```python
from build123d import *

# Parameters (mm, degrees)
SKETCH1_W           = 48
SKETCH1_H           = 53
BOSS_EXTRUDE1_DEPTH = 10
SKETCH2_W           = 48
SKETCH2_H           = 5.616325
BOSS_EXTRUDE2_DEPTH = 33.1917878
SKETCH4_W           = 4
SKETCH4_H           = 10
BOSS_EXTRUDE4_DEPTH = 40
SKETCH5_W           = 48
SKETCH5_H           = 10.8609375
BOSS_EXTRUDE5_DEPTH = 23.1917878
SKETCH6_W           = 48
SKETCH6_H           = 5
BOSS_EXTRUDE6_DEPTH = 42.3
SKETCH7_W           = 12.8082122
SKETCH7_H           = 16.4772625
BOSS_EXTRUDE7_DEPTH = 48
CUT_EXTRUDE1_REACH  = 84.426
SKETCH8_R           = 11.5
SKETCH8_R_2         = 2
FILLET1_R           = 10
FILLET2_R           = 4
SKETCH9_W           = 5
SKETCH9_H           = 16.4772625
BOSS_EXTRUDE9_DEPTH = 48


with BuildPart() as part:
    # Sketch1 → Boss-Extrude1 (new body)
    with BuildSketch(Plane.XY):
        with Locations((24, 26.5)):
            Rectangle(SKETCH1_W, SKETCH1_H)
    extrude(amount=BOSS_EXTRUDE1_DEPTH)

    # Sketch2 → Boss-Extrude2 (add)
    with BuildSketch(Plane(origin=(0, 0, 0), x_dir=(-1, 0, 0), z_dir=(0, 0, -1))):
        with Locations((-24, -2.8081625)):
            Rectangle(SKETCH2_W, SKETCH2_H)
    extrude(amount=-BOSS_EXTRUDE2_DEPTH)

    # Sketch4 → Boss-Extrude4 (add)
    with BuildSketch(Plane.XY.offset(10)):
        with Locations((2, 48)):
            Rectangle(SKETCH4_W, SKETCH4_H)
        with Locations((46, 48)):
            Rectangle(SKETCH4_W, SKETCH4_H)
    extrude(amount=BOSS_EXTRUDE4_DEPTH)

    # Sketch5 → Boss-Extrude5 (add)
    with BuildSketch(Plane.XY.offset(10)):
        with Locations((24, 5.43046875)):
            Rectangle(SKETCH5_W, SKETCH5_H)
    extrude(amount=BOSS_EXTRUDE5_DEPTH)

    # Sketch6 → Boss-Extrude6 (add)
    with BuildSketch(Plane.XZ.offset(5.616325)):
        with Locations((24, 30.6917878)):
            Rectangle(SKETCH6_W, SKETCH6_H)
    extrude(amount=BOSS_EXTRUDE6_DEPTH)

    # Sketch7 → Boss-Extrude7 (add)
    with BuildSketch(Plane.ZY):
        with Locations((-6.4041061, 2.62230625)):
            Rectangle(SKETCH7_W, SKETCH7_H)
    extrude(amount=-BOSS_EXTRUDE7_DEPTH)

    # Sketch8 → Cut-Extrude1 (cut, up to next)
    with BuildSketch(Plane(origin=(0, 0, 28.1917878), x_dir=(-1, 0, 0), z_dir=(0, 0, -1)), mode=Mode.PRIVATE) as cut_extrude1_sk1:
        with Locations((-24, -26.616325)):
            Circle(SKETCH8_R)
    cut_extrude1_tool1 = extrude(cut_extrude1_sk1.sketch, amount=-CUT_EXTRUDE1_REACH, mode=Mode.PRIVATE) & part.part
    # Sketch8 → Cut-Extrude1 (cut, up to next)
    with BuildSketch(Plane(origin=(0, 0, 28.1917878), x_dir=(-1, 0, 0), z_dir=(0, 0, -1)), mode=Mode.PRIVATE) as cut_extrude1_sk2:
        with Locations((-39.5, -11.116325)):
            Circle(SKETCH8_R_2)
    cut_extrude1_tool2 = extrude(cut_extrude1_sk2.sketch, amount=-CUT_EXTRUDE1_REACH, mode=Mode.PRIVATE) & part.part
    # Sketch8 → Cut-Extrude1 (cut, up to next)
    with BuildSketch(Plane(origin=(0, 0, 28.1917878), x_dir=(-1, 0, 0), z_dir=(0, 0, -1)), mode=Mode.PRIVATE) as cut_extrude1_sk3:
        with Locations((-39.5, -42.116325)):
            Circle(SKETCH8_R_2)
    cut_extrude1_tool3 = extrude(cut_extrude1_sk3.sketch, amount=-CUT_EXTRUDE1_REACH, mode=Mode.PRIVATE) & part.part
    # Sketch8 → Cut-Extrude1 (cut, up to next)
    with BuildSketch(Plane(origin=(0, 0, 28.1917878), x_dir=(-1, 0, 0), z_dir=(0, 0, -1)), mode=Mode.PRIVATE) as cut_extrude1_sk4:
        with Locations((-8.5, -11.116325)):
            Circle(SKETCH8_R_2)
    cut_extrude1_tool4 = extrude(cut_extrude1_sk4.sketch, amount=-CUT_EXTRUDE1_REACH, mode=Mode.PRIVATE) & part.part
    # Sketch8 → Cut-Extrude1 (cut, up to next)
    with BuildSketch(Plane(origin=(0, 0, 28.1917878), x_dir=(-1, 0, 0), z_dir=(0, 0, -1)), mode=Mode.PRIVATE) as cut_extrude1_sk5:
        with Locations((-8.5, -42.116325)):
            Circle(SKETCH8_R_2)
    cut_extrude1_tool5 = extrude(cut_extrude1_sk5.sketch, amount=-CUT_EXTRUDE1_REACH, mode=Mode.PRIVATE) & part.part
    add(cut_extrude1_tool1.solids().sort_by_distance((24, -26.616325, 28.191788))[0], mode=Mode.SUBTRACT)
    add(cut_extrude1_tool2.solids().sort_by_distance((39.5, -11.116325, 28.191788))[0], mode=Mode.SUBTRACT)
    add(cut_extrude1_tool3.solids().sort_by_distance((39.5, -42.116325, 28.191788))[0], mode=Mode.SUBTRACT)
    add(cut_extrude1_tool4.solids().sort_by_distance((8.5, -11.116325, 28.191788))[0], mode=Mode.SUBTRACT)
    add(cut_extrude1_tool5.solids().sort_by_distance((8.5, -42.116325, 28.191788))[0], mode=Mode.SUBTRACT)

    # Fillet1
    fillet1_edges = [part.edges().sort_by_distance(p)[0] for p in [
        (24, 10.8609375, 0),
    ]]
    fillet(fillet1_edges, radius=FILLET1_R)

    # Fillet2
    fillet2_edges = [part.edges().sort_by_distance(p)[0] for p in [
        (2, 43, 10),
        (46, 43, 10),
    ]]
    fillet(fillet2_edges, radius=FILLET2_R)

    # Sketch9 → Boss-Extrude9 (add)
    with BuildSketch(Plane(origin=(48, 0, 0), x_dir=(0, 0, -1), z_dir=(1, 0, 0))):
        with Locations((15.3082122, 2.62230625)):
            Rectangle(SKETCH9_W, SKETCH9_H)
    extrude(amount=-BOSS_EXTRUDE9_DEPTH)


solid = part.part
```
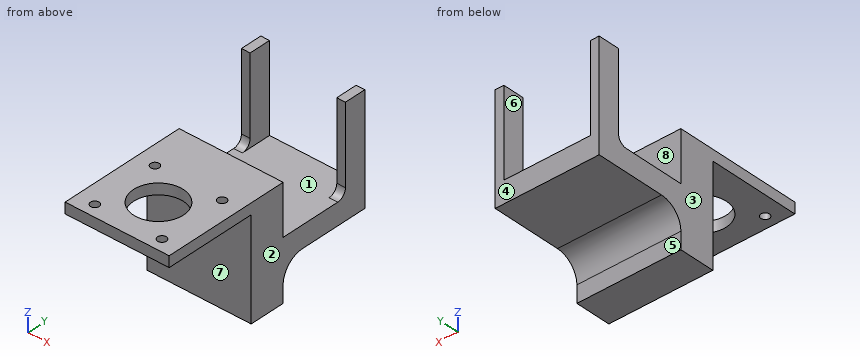
Geometry: final body of the model. Coordinates: model frame, mm. Face numbers are marked on the shaded views. A direction names the side the tool comes from. Coordinates: 2 decimals unless noted, no trailing zeros. Order: outer loops, then holes, each group sorted by start corner. A loop starts at its lowest first (then second) coordinate and runs counter-clockwise, first axis right, second up. Notation, with made-up numbers: M 34.5,-24 L 58.5,-24 A29 cw 58.5,12 Z; hole C 40,57.25 d5. An arc over 180 degrees is marked long. Answer in a Markdown table with one row per item. Add a question column.
Q1. Section query D-D on y = -28. Return the cut outline in (x, z), and give its area (3 significant figures).
Q2. Section query C-C on x = 8.5. Return the cut outline in (y, z), and give its area (3 significant figures).
Q3. Section query B-B on z = 29.5. Return the cut outline in (x, y), and give its area (3 significant figures).
Q4. Mould query, pull axis X, two halves, no side actions, for the marked faces 1, 2, 3 and 4. Classes: released by +X, released by -X, zero draft, split by the parting line, or undercut.
Q5. Line query: L1, parallel to Y at x = 8.5, z = 31.95; L2, parallel to X at y = 44.5, z = 27; L3, parallel to Y at x = 39, z = 31. Output: solid intervals per line, ascending.
Q6. Contact query for flat-ended pins moving along their axis: P1, Ø6.5, axis at x = 39.5, y = -11.12, coming from the -Z side; P2, Ø1.5, axis at x = 34, y = 38, coming from the -Z side; P3, Ø2.5, axis at x = 8.5, y = -42.12, coming from the +Z side; P4, Ø4.5, axis at x = 39.5, y = -42.12, coming from the +Z side. Output: stop coordinate, or through.
Q7. Reachability of the marked faces 5, 6, 7 and 8 from +Z, -Z, +X, -X, +Y, -Y: full face, straight path, thin tool, end or side. Return the list, or none.
Q8. Section query A-A on x = 24. Return the cut outline in (y, z).
Completed:
| question | item | result |
|---|---|---|
| 1 | outline | M 0,28.19 L 12.58,28.19 L 12.58,33.19 L 0,33.19 Z; M 35.42,28.19 L 48,28.19 L 48,33.19 L 35.42,33.19 Z |
| 1 | area | 126 mm2 |
| 2 | outline | M -47.92,28.19 L -44.12,28.19 L -44.12,33.19 L -47.92,33.19 Z; M -40.12,28.19 L -13.12,28.19 L -13.12,33.19 L -40.12,33.19 Z; M -9.12,28.19 L -5.62,28.19 L -5.62,-17.81 L 10.86,-17.81 L 10.86,-10 A10 cw 20.86,0 L 53,0 L 53,10 L 10.86,10 L 10.86,33.19 L -9.12,33.19 Z |
| 2 | area | 1,450 mm2 |
| 3 | outline | M 0,-47.92 L 48,-47.92 L 48,10.86 L 0,10.86 Z; M 0,43 L 4,43 L 4,53 L 0,53 Z; M 44,43 L 48,43 L 48,53 L 44,53 Z; hole C 8.5,-42.12 d4; hole C 8.5,-11.12 d4; hole C 24,-26.62 d23; hole C 39.5,-42.12 d4; hole C 39.5,-11.12 d4 |
| 3 | area | 2,440 mm2 |
| 4 | face 1 | undercut |
| 4 | face 2 | released by +X |
| 4 | face 3 | released by -X |
| 4 | face 4 | zero draft |
| 5 | L1 | y = -47.92 to -44.12, -40.12 to -13.12, -9.12 to 10.86 |
| 5 | L2 | x = 0 to 4, 44 to 48 |
| 5 | L3 | y = -47.92 to -44.05, -40.18 to -13.05, -9.18 to 10.86 |
| 6 | P1 | stops at z = 28.19 |
| 6 | P2 | stops at z = 0 |
| 6 | P3 | passes through |
| 6 | P4 | stops at z = 33.19 |
| 7 | face 5 | -Z, +X, -X, +Y |
| 7 | face 6 | +Z, +Y |
| 7 | face 7 | -Z, +X, -X, -Y |
| 7 | face 8 | +Z, +X, -X |
| 8 | outline | M -47.92,28.19 L -38.12,28.19 L -38.12,33.19 L -47.92,33.19 Z; M -15.12,28.19 L -5.62,28.19 L -5.62,-17.81 L 10.86,-17.81 L 10.86,-10 A10 cw 20.86,0 L 53,0 L 53,10 L 10.86,10 L 10.86,33.19 L -15.12,33.19 Z |
